Could you check a few things on this model? Use its own coordinates, in mm. Face numbers are marked on the shaded views. A direction names the side the tool comes from. Give positions to 0.01 mm unless a question says otherwise; leave off trailing zeros. Loops run counter-clockwise (first coordinate to the right, second up) from the corner with the lowest first, then second, coordinate; pieces in that order, holes last. Notation, with made-up numbers: (21, 62) - (80, 62) arc R21 cw to (80, 93) - close; hole circle Ø9 at (42, 76.5). An arc over 180 degrees is marked (long way). One line per item, written item: value. Start each with the question number.
Q1. I'm going to push flat-ended pins straight in: P1, Ø8, axis at y = 11, z = -59, coming from the -X side; P2, Ø4, axis at x = 7, y = 12.5, coming from the +Z side; P3, Ø12, axis at x = -38.5, y = 7, coming from the +Z side. Where does each tip first touch, or does it pass through?
Q2. For the marked faces 1 and 2, which set-ups out of +Z, -Z, +X, -X, +Y, -Y let a thin tool reach every point of the face, with its end or its side?
Q3. I want a section at C-C (y = 22.25). Count the separate pieces of the cut face and the enclosed holes in it, then the cut area to 3 significant figures.
Q4. If we mould it in two halves opening along Z, with no side actions, what happens to the marked faces 3, 4 and 5? For each: released by +Z, released by -Z, zero draft, split by the parting line, or undercut.
Q5. I want a section at D-D (x = 21). Please give me the cut outline in (y, z).
Q6. I want a section at A-A (z = -50.8). Please give me the cut outline in (x, y), then the cut area to 3 significant figures.
Q7. I want a section at B-B (x = 0). Please give me the cut outline in (y, z), then the cut area to 3 significant figures.
Q8. If I drill on line 1 (Z direction, x = 0, y = 18.75); line 2 (X direction, y = 12, z = -0.5); line 3 (X direction, y = 12.25, z = 33), over which ranges is the centre line in solid material (lowest first)? Write a range as from..to.
```python
from build123d import *

# Parameters (mm, degrees)
SKETCH1_R           = 63.5
SKETCH1_R_2         = 29.083
SKETCH1_R_3         = 6.35
BOSS_EXTRUDE1_DEPTH = 25.4
CUT_EXTRUDE3_DEPTH  = 6.35
CIRPATTERN1_COUNT   = 3
SKETCH5_R           = 3.302
CUT_EXTRUDE4_DEPTH  = 26.4
CIRPATTERN2_COUNT   = 3


with BuildPart() as part:
    # Sketch1 → Boss-Extrude1 (new body)
    with BuildSketch(Plane(origin=(0, 0, 0), x_dir=(1, 0, 0), z_dir=(0, 1, 0))):
        Circle(SKETCH1_R)
        Circle(SKETCH1_R_2, mode=Mode.SUBTRACT)
        with Locations((0, 50.8)):
            Circle(SKETCH1_R_3, mode=Mode.SUBTRACT)
        with Locations((43.994090512, -25.4)):
            Circle(SKETCH1_R_3, mode=Mode.SUBTRACT)
        with Locations((-43.994090512, -25.4)):
            Circle(SKETCH1_R_3, mode=Mode.SUBTRACT)
    extrude(amount=BOSS_EXTRUDE1_DEPTH)

    # Sketch4 → Cut-Extrude3 (cut, symmetric)
    with BuildSketch(Plane(origin=(0, 0, 0), x_dir=(0, 0, -1), z_dir=(1, 0, 0))):
        Polygon((63.5, 0), (63.5, 6.35), (53.360319725, 23.912441409), (53.360319725, 0), align=None)
    cut_extrude3 = extrude(amount=CUT_EXTRUDE3_DEPTH, both=True, mode=Mode.SUBTRACT)

    # CirPattern1: Cut-Extrude3 ×3 about axis
    cirpattern1_axis = Axis((0, 0, 0), (0, 1, 0))
    for i in range(1, CIRPATTERN1_COUNT):
        add(cut_extrude3.rotate(cirpattern1_axis, i * 360 / CIRPATTERN1_COUNT), mode=Mode.SUBTRACT)

    # Sketch5 → Cut-Extrude4 (cut, through all)
    with BuildSketch(Plane(origin=(0, 25.4, 0), x_dir=(1, 0, 0), z_dir=(0, 1, 0))):
        with Locations((-43.229109276, 14.884976022)):
            Circle(SKETCH5_R)
    cut_extrude4 = extrude(amount=-CUT_EXTRUDE4_DEPTH, mode=Mode.SUBTRACT)

    # CirPattern2: Cut-Extrude4 ×3 about axis
    cirpattern2_axis = Axis((0, 0, 0), (0, 1, 0))
    for i in range(1, CIRPATTERN2_COUNT):
        add(cut_extrude4.rotate(cirpattern2_axis, i * 360 / CIRPATTERN2_COUNT), mode=Mode.SUBTRACT)


solid = part.part
```
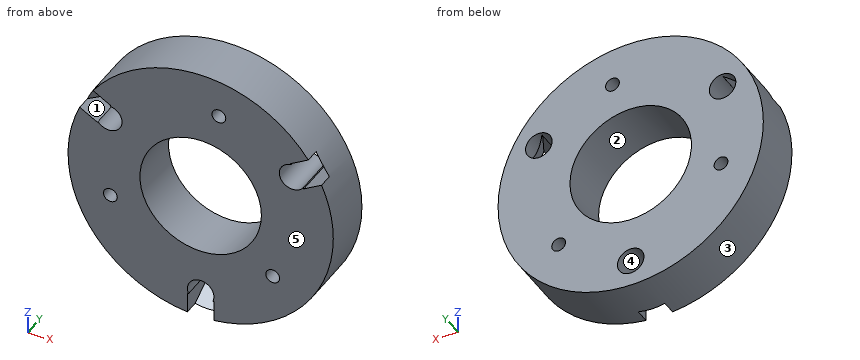
Worked answers:
1. P1: stops at x = -31.74
1. P2: stops at z = 63.3
1. P3: stops at z = 54.55
2. face 1: -Y
2. face 2: +Y, -Y
3. separate pieces: 1
3. enclosed holes: 7
3. area: 9,520 mm²
4. face 3: split by the parting line
4. face 4: undercut
4. face 5: zero draft
5. outline: (0, -59.93) - (25.4, -59.93) - (25.4, -20.12) - (0, -20.12) - close; (0, 20.12) - (25.4, 20.12) - (25.4, 59.93) - (0, 59.93) - close
6. outline: (-38.1, 0) - (-6.35, 0) - (-6.35, 25.4) - (-38.1, 25.4) - close; (6.35, 0) - (38.1, 0) - (38.1, 25.4) - (6.35, 25.4) - close
6. area: 1,610 mm²
7. outline: (0, -44.45) - (25.4, -44.45) - (25.4, -29.08) - (0, -29.08) - close; (0, 29.08) - (25.4, 29.08) - (25.4, 63.5) - (0, 63.5) - close; (6.35, -63.5) - (25.4, -63.5) - (25.4, -57.15) - (17.35, -57.15) - close
7. area: 1,350 mm²
8. line 1: z = -63.5..-57.15, -44.45..-29.08, 29.08..63.5
8. line 2: x = -63.5..-29.08, 29.08..63.5
8. line 3: x = -54.25..-50.34, -44.46..44.46, 50.34..54.25
